```python
from build123d import *

# Parameters (mm, degrees)
PLATE_BODY_DEPTH     = 2
SKETCH2_R            = 4.1
SHAFT_BEARINGS_DEPTH = 3
SLOT_DEPTH           = 3
SKETCH5_R            = 1.25
BOLT_HOLES_DEPTH     = 3
SKETCH6_W            = 0.5
SKETCH6_H            = 40
CUT_EXTRUDE1_DEPTH   = 3
SKETCH8_W            = 3
SKETCH8_H            = 5
FINGER_JOINTS_DEPTH  = 2
F_1MM_FILLETS_R      = 1


with BuildPart() as part:
    # Sketch1 → plate_body (new body)
    with BuildSketch(Plane.XY):
        Polygon((0, 40), (0, 0), (40, 0), (40, -5), (44, -5), (44, -11), (50, -11), (50, -51), (76.5, -51), (76.5, 10), (50, 10), (50, 40), align=None)
    extrude(amount=PLATE_BODY_DEPTH)

    # Sketch2 → shaft_bearings (cut, through all)
    with BuildSketch(Plane.XY.offset(2)):
        with Locations((6, 20)):
            Circle(SKETCH2_R)
        with Locations((44, 20)):
            Circle(SKETCH2_R)
    extrude(amount=-SHAFT_BEARINGS_DEPTH, mode=Mode.SUBTRACT)

    # Sketch4 → slot (cut, through all)
    with BuildSketch(Plane.XY.offset(2)):
        with BuildLine():
            Line((26.75, 34), (26.75, 6))
            ThreePointArc((26.75, 6), (25, 4.25), (23.25, 6))
            Line((23.25, 6), (23.25, 34))
            ThreePointArc((23.25, 34), (25, 35.75), (26.75, 34))
        make_face()
    extrude(amount=-SLOT_DEPTH, mode=Mode.SUBTRACT)

    # Sketch5 → bolt_holes (cut, through all)
    with BuildSketch(Plane.XY.offset(2)):
        with Locations((3, 37)):
            Circle(SKETCH5_R)
        with Locations((47, 37)):
            Circle(SKETCH5_R)
        with Locations((3, 3)):
            Circle(SKETCH5_R)
        with Locations((47, 3)):
            Circle(SKETCH5_R)
    extrude(amount=-BOLT_HOLES_DEPTH, mode=Mode.SUBTRACT)

    # Sketch6 → Cut-Extrude1 (cut, through all)
    with BuildSketch(Plane.XY.offset(2)):
        with Locations((50.25, -31)):
            Rectangle(SKETCH6_W, SKETCH6_H)
    extrude(amount=-CUT_EXTRUDE1_DEPTH, mode=Mode.SUBTRACT)

    # Sketch8 → finger_joints (add)
    with BuildSketch(Plane.XY.offset(2)):
        with Locations((49, -33.5)):
            Rectangle(SKETCH8_W, SKETCH8_H)
        with Locations((49, -43.5)):
            Rectangle(SKETCH8_W, SKETCH8_H)
        with Locations((78, -43.5)):
            Rectangle(SKETCH8_W, SKETCH8_H)
        with Locations((78, -33.5)):
            Rectangle(SKETCH8_W, SKETCH8_H)
        with Locations((49, -13.5)):
            Rectangle(SKETCH8_W, SKETCH8_H)
        with Locations((49, -23.5)):
            Rectangle(SKETCH8_W, SKETCH8_H)
        with Locations((78, -23.5)):
            Rectangle(SKETCH8_W, SKETCH8_H)
        with Locations((78, -13.5)):
            Rectangle(SKETCH8_W, SKETCH8_H)
    extrude(amount=-FINGER_JOINTS_DEPTH)

    # 1mm_fillets
    f_1mm_fillets_edges = [part.edges().sort_by_distance(p)[0] for p in [
        (44, -11, 1),
        (44, -5, 1),
        (40, -5, 1),
        (40, 0, 1),
        (0, 0, 1),
        (0, 40, 1),
        (50, 40, 1),
        (50, 10, 1),
        (76.5, 10, 1),
    ]]
    fillet(f_1mm_fillets_edges, radius=F_1MM_FILLETS_R)


solid = part.part
```
Can you work these out from the model? Positions are in its coordinate system, mm. A direction names the side the tool comes from. Coordinates: 2 decimals unless noted, no trailing zeros. Order: outer loops, then holes, each group sorted by start corner. A loop starts at its lowest first (then second) coordinate and runs counter-clockwise, first axis right, second up.
1. For faces 5 (the face through (20, 0, 1)), 6 (the face through (49, -41, 1)), 7 (the face through (76.5, -19, 1)), 8 (the face through (79.5, -44, 1)), 9 (the face through (78, -46, 1)), which set-ups out of +Z, -Z, +X, -X, +Y, -Y let a thin tool reach every point of the face, with its end or its side?
2. I need wall thicknesses on line 1 (Y direction, x = 3, z = 0.5); line 2 (X direction, y = 8.5, z = 1.4); line 3 (Y direction, x = 6, z = 0.95). Which ranges of each line are inside material? Lowest first, please.
3. If we section it at B-B (x = 3): Please give me the cut outline in (y, z).
4. I'm going to push flat-ended pins straight in: pin 1 (1 mm diameter, centred on x = 78, z = 1.5, fed in from +Y); pin 2 (0.6 mm diameter, centred on y = -18.5, z = 1, fed in from -X); pin 3 (0.6 mm diameter, centred on y = -24, z = 1, fed in from -X). Where does each tip first touch, or does it pass through?
5. If we section it at D-D (y = 3): Please give me the cut outline in (x, z).
6. Thinking about a two-plate mould opening in X: for faces 1 (the face through (76.5, -39, 1)), 2 (the face through (3.577, 35.891, 1.014)), 3 (the face through (25.04, 4.25, 1.01)), 4 (the face through (46, -11, 1)), which applies, +X half, -X half, draft (parallel to the pull), parting line (faces both ways), or undercut?
7. If we section it at A-A (y = 37): Please give me the cut outline in (x, z), then the cut area to 3 significant figures.
8. If we section it at C-C (z = 0.95): Give the number of separate pieces and of enclosed holes in the cut face, then the cut area to 3 significant figures.
Entries:
1. face 5: +Z, -Z, -X, -Y
1. face 6: +Z, -Z, -X
1. face 7: +Z, -Z, +X
1. face 8: +Z, -Z, +X, +Y, -Y
1. face 9: +Z, -Z, +X, -Y
2. line 1: y = 0 to 1.75, 4.25 to 17.21, 22.79 to 35.75, 38.25 to 40
2. line 2: x = 0 to 23.25, 26.75 to 76.5
2. line 3: y = 0 to 15.9, 24.1 to 40
3. outline: (0, 0) - (1.75, 0) - (1.75, 2) - (0, 2) - close; (4.25, 0) - (17.21, 0) - (17.21, 2) - (4.25, 2) - close; (22.79, 0) - (35.75, 0) - (35.75, 2) - (22.79, 2) - close; (38.25, 0) - (40, 0) - (40, 2) - (38.25, 2) - close
4. pin 1: stops at y = -11
4. pin 2: stops at x = 50.5
4. pin 3: stops at x = 47.5
5. outline: (0, 0) - (1.75, 0) - (1.75, 2) - (0, 2) - close; (4.25, 0) - (45.75, 0) - (45.75, 2) - (4.25, 2) - close; (48.25, 0) - (76.5, 0) - (76.5, 2) - (48.25, 2) - close
6. face 1: +X half
6. face 2: undercut
6. face 3: undercut
6. face 4: draft
7. outline: (0, 0) - (1.75, 0) - (1.75, 2) - (0, 2) - close; (4.25, 0) - (45.75, 0) - (45.75, 2) - (4.25, 2) - close; (48.25, 0) - (50, 0) - (50, 2) - (48.25, 2) - close
7. area: 90.0 mm2
8. separate pieces: 1
8. enclosed holes: 7
8. area: 3,570 mm2
